Geometry: see drawing. Coordinates: mm, zero at the bounding-box minimum. Give positions to 0.01 mm unless a question says otherwise; leave off trailing zeros. Write each loop counter-clockwise with the first axis right and the second up, starting at its lowest first coordinate (ties: lowest second). Pieces come first, ordered by that corner, then holes. Notation, with made-up numbers: (17, 13) - (52, 13) arc R16 cw to (52, 24) - close; hole circle Ø7 at (12.25, 48.25). An arc over 180 degrees is marked (long way). Return JSON: item names as keys, results as strings.
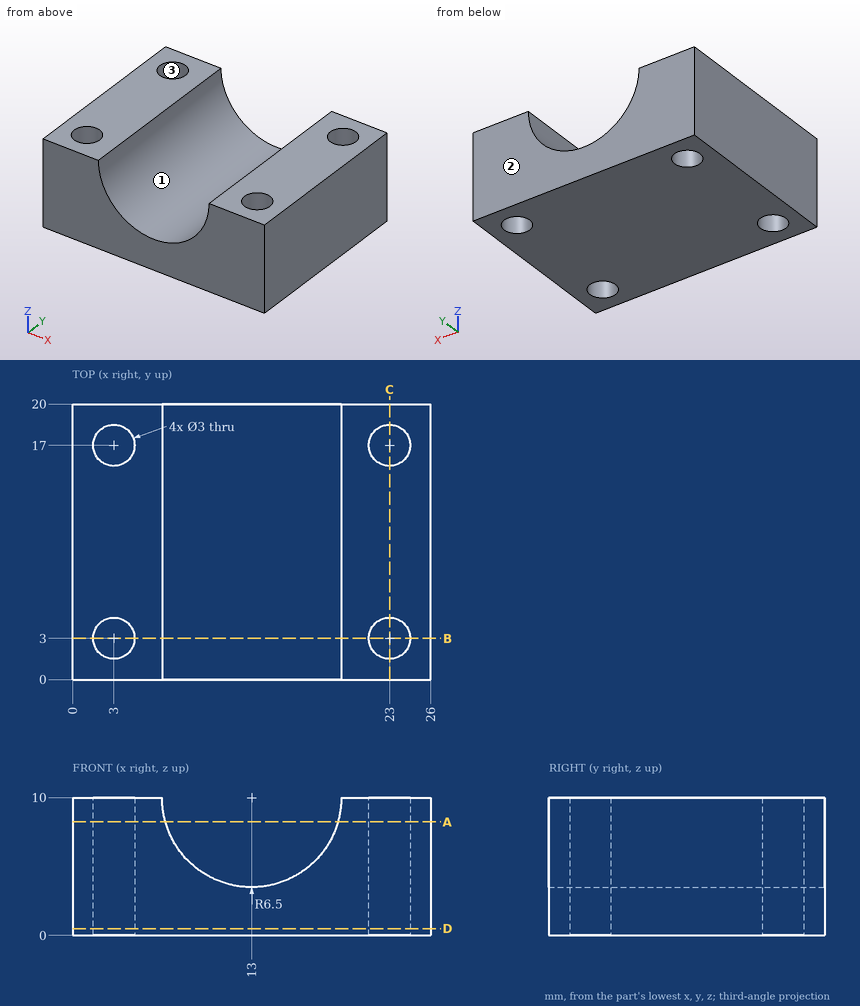
Q1. Section query A-A, the plane z = 8.25. Return the cut outline in (x, y), plus the area to 3 significant figures.
Answer key:
{"outline": "(0, 0) - (6.74, 0) - (6.74, 20) - (0, 20) - close; (19.26, 0) - (26, 0) - (26, 20) - (19.26, 20) - close; hole circle Ø3 at (3, 3); hole circle Ø3 at (3, 17); hole circle Ø3 at (23, 3); hole circle Ø3 at (23, 17)", "area": "241 mm^2"}
Q2. Section query B-B, the plane y = 3. Return the cut outline in (x, z).
Answer key:
{"outline": "(0, 0) - (1.5, 0) - (1.5, 10) - (0, 10) - close; (4.5, 0) - (21.5, 0) - (21.5, 10) - (19.5, 10) arc R6.5 cw to (6.5, 10) - (4.5, 10) - close; (24.5, 0) - (26, 0) - (26, 10) - (24.5, 10) - close"}
Q3. Section query C-C, the plane x = 23. Return the cut outline in (y, z).
Answer key:
{"outline": "(0, 0) - (1.5, 0) - (1.5, 10) - (0, 10) - close; (4.5, 0) - (15.5, 0) - (15.5, 10) - (4.5, 10) - close; (18.5, 0) - (20, 0) - (20, 10) - (18.5, 10) - close"}
Q4. Material intervals for probe 1 along Y at (x, z) = (3, 3); probe 2 along Y at (x, z) = (22.5, 4); probe 3 along X at (y, z) = (4.25, 1.5), sorted ascending. Write a range as [from, to].
Answer key:
{"probe 1": "y = [0, 1.5], [4.5, 15.5], [18.5, 20]", "probe 2": "y = [0, 1.59], [4.41, 15.59], [18.41, 20]", "probe 3": "x = [0, 2.17], [3.83, 22.17], [23.83, 26]"}
Q5. Pin query (flat end, axial travel): P1, Ø10, axis at x = 13, y = 7.5, coming from the +Z side; P2, Ø4, axis at x = 23, y = 17, coming from the +Z side. Return the tip coordinate at first contact, or that it passes through.
Answer key:
{"P1": "stops at z = 5.85", "P2": "stops at z = 10"}
Q6. Section query D-D, the plane z = 0.5. Return the cut outline in (x, y), plus the area to 3 significant figures.
Answer key:
{"outline": "(0, 0) - (26, 0) - (26, 20) - (0, 20) - close; hole circle Ø3 at (3, 3); hole circle Ø3 at (3, 17); hole circle Ø3 at (23, 3); hole circle Ø3 at (23, 17)", "area": "492 mm^2"}
Q7. Mould query, pull axis Y, two halves, no side actions, for the marked faces 1, 2 and 3. Classes: pulls with the +Y half, pulls with the -Y half, needs draft (parallel to the pull), parting line crosses it, or undercut.
Answer key:
{"face 1": "needs draft", "face 2": "pulls with the +Y half", "face 3": "undercut"}
